Geometry check sheet. Reference: the model listing, model coordinates, mm. Round coordinates to 2 decimals unless told otherwise and drop trailing zeros. Write each loop counter-clockwise with the first axis right and the second up, starting at its lowest first coordinate (ties: lowest second). Pieces come first, ordered by that corner, then holes. Notation, with made-up numbers: (-18.75, -34) -> (24.25, -34) arc R20 ccw to (24.25, -7) -> close; hole circle Ø8 at (-18, 21.5). An arc over 180 degrees is marked (long way). Use a Markdown table: item, result.
```python
from build123d import *

# Parameters (mm, degrees)
SKETCH1_W                     = 139.7
SKETCH1_H                     = 50.8
BOSS_EXTRUDE1_DEPTH           = 38.1
F_0_4IN_DIAMETER_HOLE_ZAXIS_D = 10.16
F_0_4IN_DIAMETER_HOLE_YAXIS_D = 10.16


with BuildPart() as part:
    # Sketch1 → Boss-Extrude1 (new, symmetric)
    with BuildSketch(Plane.XY):
        Rectangle(SKETCH1_W, SKETCH1_H)
    extrude(amount=BOSS_EXTRUDE1_DEPTH, both=True)

    # 0.4in Diameter Hole zaxis (through all)
    with Locations(Plane.XY.offset(38.1)):
        with Locations((46.99, 9.652), (44.45, -9.652)):
            f_0_4in_diameter_hole_zaxis = Hole(F_0_4IN_DIAMETER_HOLE_ZAXIS_D / 2)

    # Mirror1: 0.4in Diameter Hole zaxis across plane
    add(f_0_4in_diameter_hole_zaxis.mirror(Plane(origin=(0, 0, 0), x_dir=(0, 0, 1), z_dir=(1, 0, 0))), mode=Mode.SUBTRACT)

    # 0.4in Diameter Hole yaxis (through all)
    with Locations(Plane(origin=(0, 25.4, 0), x_dir=(1, 0, 0), z_dir=(0, 1, 0))):
        with Locations((-25.4, 25.4), (-25.4, -25.4), (25.4, -25.4), (25.4, 25.4)):
            Hole(F_0_4IN_DIAMETER_HOLE_YAXIS_D / 2)


solid = part.part
```
(1) Release check for a two-part mould opening along X. For faces 1 (the face through (-1, 25.4, 1)), 2 (the face through (29.144, -0.356, -28.833)), 3 (the face through (69.85, 0, 1)) record: +X half, -X half, draft (parallel to the pull), parting line (faces both ways), or undercut.
A:
| item | result |
|---|---|
| face 1 | draft |
| face 2 | undercut |
| face 3 | +X half |
(2) Section check C-C on x = -46.99. Record the cut outline in (y, z).
A:
| item | result |
|---|---|
| outline | (-25.4, -38.1) -> (-14.05, -38.1) -> (-14.05, 38.1) -> (-25.4, 38.1) -> close; (-5.25, -38.1) -> (4.57, -38.1) -> (4.57, 38.1) -> (-5.25, 38.1) -> close; (14.73, -38.1) -> (25.4, -38.1) -> (25.4, 38.1) -> (14.73, 38.1) -> close |
(3) Section check A-A on z = 22.5. Record the cut outline in (x, y), plus the area to 3 significant figures.
A:
| item | result |
|---|---|
| outline | (-69.85, -25.4) -> (-29.57, -25.4) -> (-29.57, 25.4) -> (-69.85, 25.4) -> close; (-21.23, -25.4) -> (21.23, -25.4) -> (21.23, 25.4) -> (-21.23, 25.4) -> close; (29.57, -25.4) -> (69.85, -25.4) -> (69.85, 25.4) -> (29.57, 25.4) -> close; hole circle Ø10.16 at (-46.99, 9.65); hole circle Ø10.16 at (-44.45, -9.65); hole circle Ø10.16 at (44.45, -9.65); hole circle Ø10.16 at (46.99, 9.65) |
| area | 5,920 mm2 |
(4) Section check D-D on y = 1.5. Record the cut outline in (x, z), plus the area to 3 significant figures.
A:
| item | result |
|---|---|
| outline | (-69.85, -38.1) -> (69.85, -38.1) -> (69.85, 38.1) -> (-69.85, 38.1) -> close; hole circle Ø10.16 at (-25.4, -25.4); hole circle Ø10.16 at (-25.4, 25.4); hole circle Ø10.16 at (25.4, -25.4); hole circle Ø10.16 at (25.4, 25.4) |
| area | 10,300 mm2 |
(5) Thickness scan on line 1 (X direction, y = -2, z = -25); line 2 (X direction, y = -10, z = -25.5); line 3 (Z direction, x = 25.4, y = -7). Record the ranges inside material, lowest first.
A:
| item | result |
|---|---|
| line 1 | x = -69.85 to -30.46, -20.34 to 20.34, 30.46 to 69.85 |
| line 2 | x = -69.85 to -49.52, -39.38 to -30.48, -20.32 to 20.32, 30.48 to 39.38, 49.52 to 69.85 |
| line 3 | z = -38.1 to -30.48, -20.32 to 20.32, 30.48 to 38.1 |
(6) Section check B-B on y = 11.5. Record the cut outline in (x, z), plus the area to 3 significant figures.
A:
| item | result |
|---|---|
| outline | (-69.85, -38.1) -> (-51.72, -38.1) -> (-51.72, 38.1) -> (-69.85, 38.1) -> close; (-42.26, -38.1) -> (42.26, -38.1) -> (42.26, 38.1) -> (-42.26, 38.1) -> close; (51.72, -38.1) -> (69.85, -38.1) -> (69.85, 38.1) -> (51.72, 38.1) -> close; hole circle Ø10.16 at (-25.4, -25.4); hole circle Ø10.16 at (-25.4, 25.4); hole circle Ø10.16 at (25.4, -25.4); hole circle Ø10.16 at (25.4, 25.4) |
| area | 8,880 mm2 |
